Design review of the part built by this model. Coordinates are the model's own, in mm. Face numbers are marked on the shaded views. Coordinates: 2 decimals unless noted, no trailing zeros. Write each loop counter-clockwise with the first axis right and the second up, starting at its lowest first coordinate (ties: lowest second). Pieces come first, ordered by that corner, then holes. Notation, with made-up numbers: (1, 65) - (44, 65) arc R28 cw to (44, 96) - close; hole circle Ø3 at (16, 17). An arc over 180 degrees is marked (long way). Use a Markdown table: item, result.
from build123d import *

# Parameters (mm, degrees)
SKETCH_1_W         = 20
SKETCH_1_H         = 10
EXTRUDE_1_DEPTH    = 4
M3X0_51_AT_2_COUNT = 2
M3X0_51_AT_2_PITCH = 9


with BuildPart() as part:
    # Эскиз1 → Бобышка-Вытянуть1 (new body)
    with BuildSketch(Plane.XY):
        Rectangle(SKETCH_1_W, SKETCH_1_H)
    extrude(amount=EXTRUDE_1_DEPTH)

    # Эскиз2 → Отверстие обработанное метчиком M3x0.51 (revolve, cut)
    with BuildSketch(Plane(origin=(-4.5, 0, 4), x_dir=(0, -1, 0), z_dir=(1, 0, 0))):
        Polygon((0, 0), (0, 4), (1.65, 4), (1.25, 3.6), (1.25, 0.4), (1.65, 0), align=None)
    m3x0_51 = revolve(axis=Axis((-4.5, 0, 10.35), (0, 0, -1)), mode=Mode.SUBTRACT)

    # Отверстие обработанное метчиком M3x0.51 at 2: Отверстие обработанное метчиком M3x0.51 ×2
    with Locations(*[(i * M3X0_51_AT_2_PITCH, 0, 0) for i in range(1, M3X0_51_AT_2_COUNT)]):
        add(m3x0_51, mode=Mode.SUBTRACT)


solid = part.part
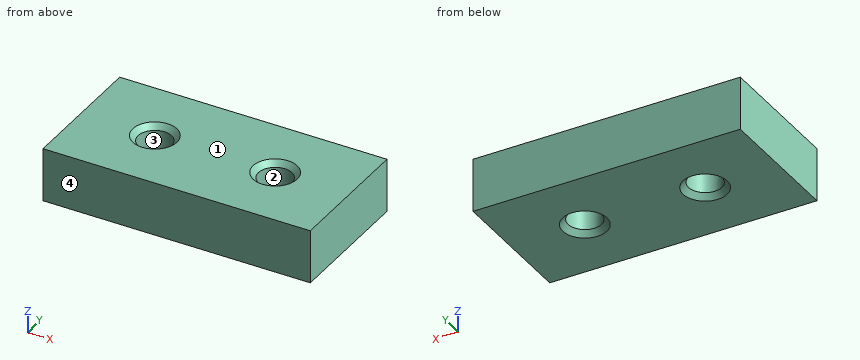
(1) Take a section at A-A on y = 0. Write out the cut boundary in (x, z), and give its area (3 significant figures).
Determined:
| item | result |
|---|---|
| outline | (-10, 0) - (-6.15, 0) - (-5.75, 0.4) - (-5.75, 3.6) - (-6.15, 4) - (-10, 4) - close; (-3.25, 0.4) - (-2.85, 0) - (2.85, 0) - (3.25, 0.4) - (3.25, 3.6) - (2.85, 4) - (-2.85, 4) - (-3.25, 3.6) - close; (5.75, 0.4) - (6.15, 0) - (10, 0) - (10, 4) - (6.15, 4) - (5.75, 3.6) - close |
| area | 59.4 mm2 |
(2) For L1, parallel to X at y = 0, z = 2.85; L2, parallel to Y at x = -4.5, z = 1.9; L3, parallel to X at y = 0.5, z = 1.1, list the stretches that pass through material, from the lowest coordinate up. Write a range as from..to.
Determined:
| item | result |
|---|---|
| L1 | -10..-5.75, -3.25..3.25, 5.75..10 |
| L2 | -5..-1.25, 1.25..5 |
| L3 | -10..-5.65, -3.35..3.35, 5.65..10 |
(3) Take a section at C-C on z = 2.95. Write out the cut boundary in (x, y).
Determined:
| item | result |
|---|---|
| outline | (-10, -5) - (10, -5) - (10, 5) - (-10, 5) - close; hole circle Ø2.5 at (-4.5, 0); hole circle Ø2.5 at (4.5, 0) |
(4) Take a section at B-B on x = -4.5. Write out the cut boundary in (y, z), and give its area (3 significant figures).
Determined:
| item | result |
|---|---|
| outline | (-5, 0) - (-1.65, 0) - (-1.25, 0.4) - (-1.25, 3.6) - (-1.65, 4) - (-5, 4) - close; (1.25, 0.4) - (1.65, 0) - (5, 0) - (5, 4) - (1.65, 4) - (1.25, 3.6) - close |
| area | 29.7 mm2 |
(5) Draft analysis for pull direction Y (two halves, no side actions). For the marked faces 1, 2, 3 and 4, state which applies: +Y half, -Y half, draft (parallel to the pull), parting line (faces both ways), or undercut.
Determined:
| item | result |
|---|---|
| face 1 | draft |
| face 2 | undercut |
| face 3 | undercut |
| face 4 | -Y half |
(6) For pin 1 (3 mm diameter, centred on x = 4.5, y = 0, fed in from +Z); pin 2 (1.5 mm diameter, centred on x = -4.5, y = 0, fed in from -Z), all flat-tipped, find the tip position at first contact; note any pin that passes through.
Determined:
| item | result |
|---|---|
| pin 1 | z = 3.85 |
| pin 2 | through |
